Print and shaded views of the part. All mm, measured from the part's lowest x, y and z. A direction names the side the tool comes from. Round coordinates to 2 decimals unless told otherwise and drop trailing zeros. Loops run counter-clockwise (first coordinate to the right, second up) from the corner with the lowest first, then second, coordinate; pieces in that order, holes last. Notation, with made-up numbers: (24, -9.75) -> (67, -9.75) arc R15 ccw to (67, 3.25) -> close; hole circle Ø2 at (-38, 2.25). An arc over 180 degrees is marked (long way). Use a Markdown table: item, result.
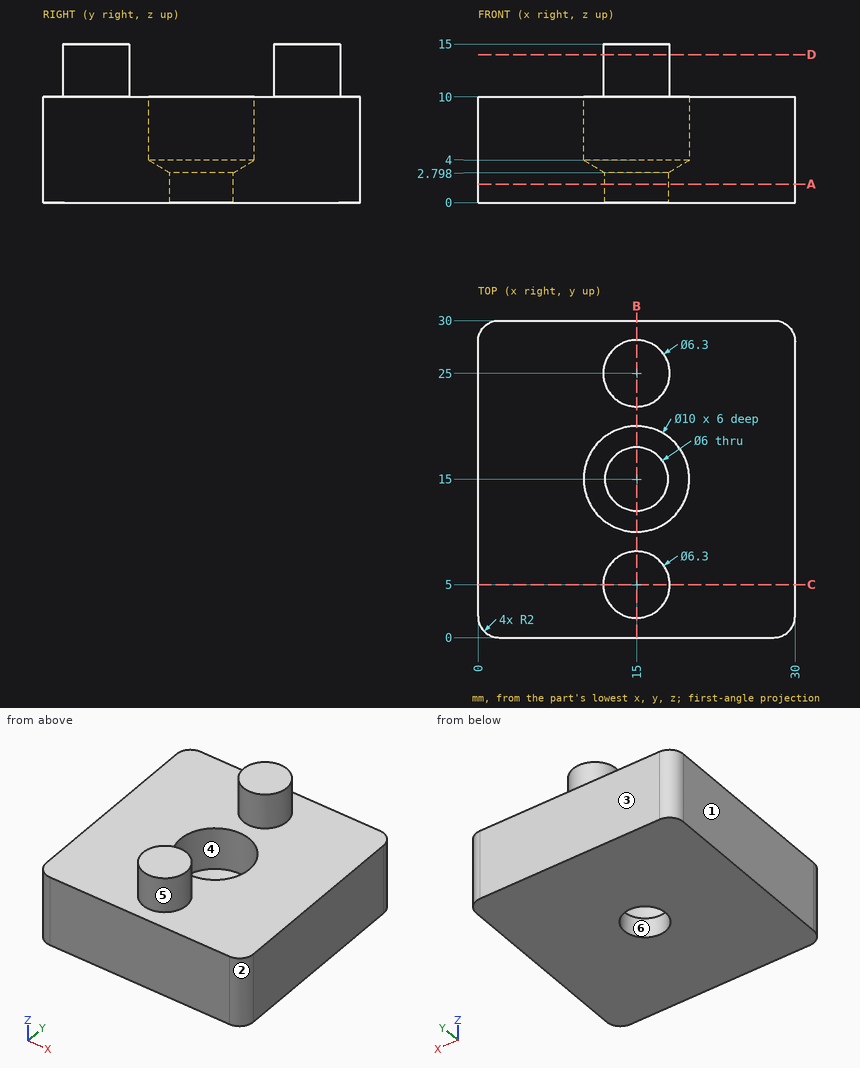
Q1. Flat gauge pins, fed straight in: pin 1 (6 mm diameter, centred on x = 14, z = 13.5, fed in from -Y); pin 2 (5 mm diameter, centred on x = 17.5, y = 16.5, fed in from +Z). Where does each tip first touch, or does it go through?
Results list:
| item | result |
|---|---|
| pin 1 | stops at y = 1.85 |
| pin 2 | stops at z = 10 |
Q2. Band-saw the part on B-B, the plane x = 15. Give the cut face in (y, z).
Results list:
| item | result |
|---|---|
| outline | (0, 0) -> (12, 0) -> (12, 2.8) -> (10, 4) -> (10, 10) -> (8.15, 10) -> (8.15, 15) -> (1.85, 15) -> (1.85, 10) -> (0, 10) -> close; (18, 0) -> (30, 0) -> (30, 10) -> (28.15, 10) -> (28.15, 15) -> (21.85, 15) -> (21.85, 10) -> (20, 10) -> (20, 4) -> (18, 2.8) -> close |
Q3. Band-saw the part on A-A, the plane z = 1.75. Give the cut face in (x, y).
Results list:
| item | result |
|---|---|
| outline | (0, 2) arc R2 ccw to (2, 0) -> (28, 0) arc R2 ccw to (30, 2) -> (30, 28) arc R2 ccw to (28, 30) -> (2, 30) arc R2 ccw to (0, 28) -> close; hole circle Ø6 at (15, 15) |
Q4. Drill centre lines: L1, parallel to Y at x = 15, z = 5.75; L2, parallel to Y at x = 15, z = 1.6; L3, parallel to Z at x = 21.25, y = 27.5. Where is each one in solid material? Low to high. Write a range as from..to.
Results list:
| item | result |
|---|---|
| L1 | y = 0..10, 20..30 |
| L2 | y = 0..12, 18..30 |
| L3 | z = 0..10 |
Q5. Band-saw the part on C-C, the plane y = 5. Give the cut face in (x, z).
Results list:
| item | result |
|---|---|
| outline | (0, 0) -> (30, 0) -> (30, 10) -> (18.15, 10) -> (18.15, 15) -> (11.85, 15) -> (11.85, 10) -> (0, 10) -> close |
Q6. Tool access for the marked faces 5 and 6: list every direction of +Z, -Z, +X, -X, +Y, -Y with a clear straight run to the whole face (end or side of a thin tool).
Results list:
| item | result |
|---|---|
| face 5 | +Z |
| face 6 | +Z, -Z |
Q7. Pull direction X, two halves, no side cores. Call the marked faces 1, 2, 3 and 4: released by +X, released by -X, zero draft, split by the parting line, or undercut.
Results list:
| item | result |
|---|---|
| face 1 | released by -X |
| face 2 | released by +X |
| face 3 | zero draft |
| face 4 | undercut |
Q8. Band-saw the part on D-D, the plane z = 14. Give the cut face in (x, y).
Results list:
| item | result |
|---|---|
| outline | circle Ø6.3 at (15, 5); circle Ø6.3 at (15, 25) |
